Check sheet for the drawn part. Datum: minimum x, y, z corner. Units: mm. Coordinates: 2 decimals unless noted, no trailing zeros. Loops run counter-clockwise (first coordinate to the right, second up) from the corner with the lowest first, then second, coordinate; pieces in that order, holes last. Notation, with made-up numbers: M 74,80 L 117,80 A29 cw 117,103 Z; hole C 49.25,-10 d5. An arc over 180 degrees is marked long. Answer in a Markdown table with one row per item. Add a question column.
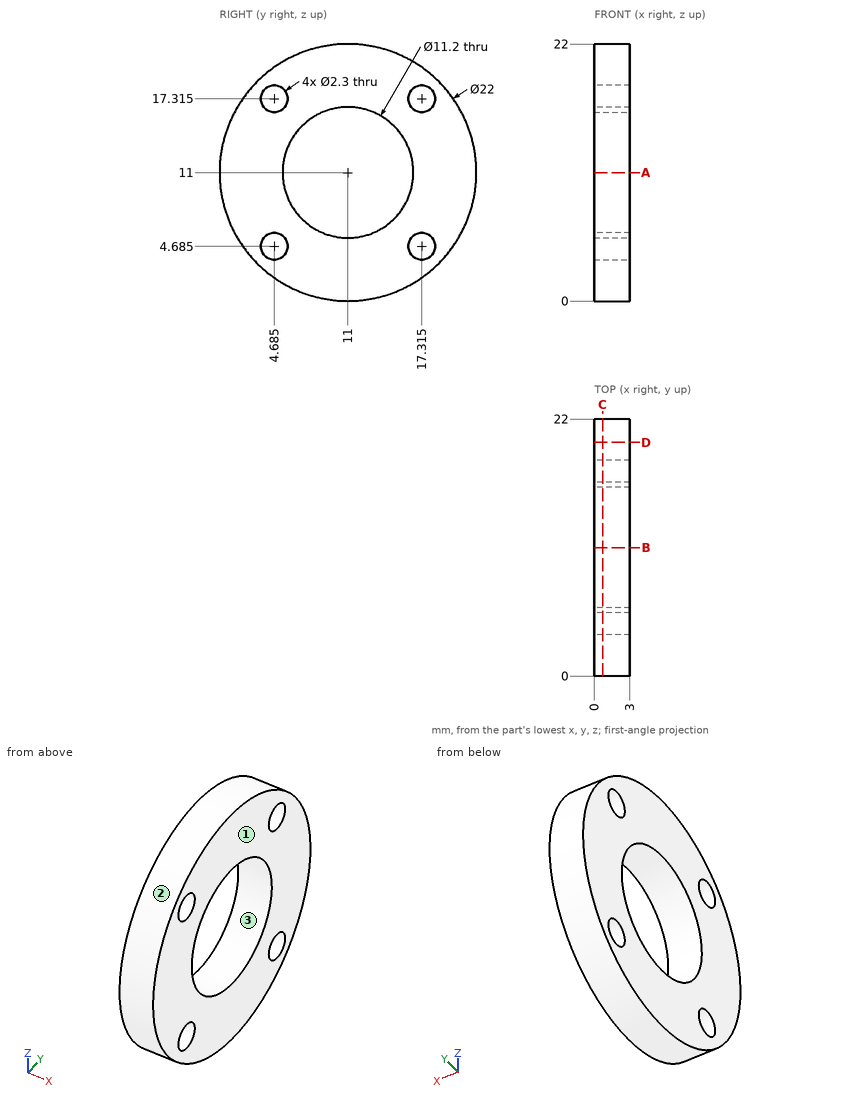
Q1. Cross-section at D-D (y = 20). Record the cut outline in (x, z) (1 decimal).
Q2. Cross-section at C-C (x = 0.7). Count the separate pieces of the cut face and the enclosed holes in it, plus the area to 3 significant figures.
Q3. Go/stop test with flat-tipped pins: pin 1 (1 mm diameter, centred on x = 2.5, z = 4, fed in from +Y) (1 decimal); pin 2 (12 mm diameter, centred on y = 11.5, z = 14.5, fed in from -X); pin 3 (1 mm diameter, centred on x = 2, z = 5, fed in from +Y) (1 decimal). Record where each tip stops, or that it passes through.
Q4. Cross-section at A-A (z = 11). Record the cut outline in (x, y).
Q5. Mould release check, pull along Y, two halves, no side actions. Record for the marked faces 1, 2 and 3: released by +Y, released by -Y, zero draft, split by the parting line, or undercut.
Q6. Thickness scan on L1, parallel to Z at x = 2.3, y = 18 (1 decimal); L2, parallel to Z at x = 2.5, y = 17; L3, parallel to Y at x = 1.7, z = 7.5. Record the ranges inside material, lowest first.
Answer key:
| question | item | result |
|---|---|---|
| 1 | outline | M 0,4.7 L 3,4.7 L 3,17.3 L 0,17.3 Z |
| 2 | separate pieces | 1 |
| 2 | enclosed holes | 5 |
| 2 | area | 265 mm^2 |
| 3 | pin 1 | y = 19.9 |
| 3 | pin 2 | x = 0 |
| 3 | pin 3 | y = 20.5 |
| 4 | outline | M 0,0 L 3,0 L 3,5.4 L 0,5.4 Z; M 0,16.6 L 3,16.6 L 3,22 L 0,22 Z |
| 5 | face 1 | zero draft |
| 5 | face 2 | split by the parting line |
| 5 | face 3 | undercut |
| 6 | L1 | 2.5 to 3.8, 5.6 to 16.4, 18.2 to 19.5 |
| 6 | L2 | 1.78 to 3.58, 5.79 to 16.21, 18.42 to 20.22 |
| 6 | L3 | 0.57 to 6.63, 15.37 to 21.43 |
